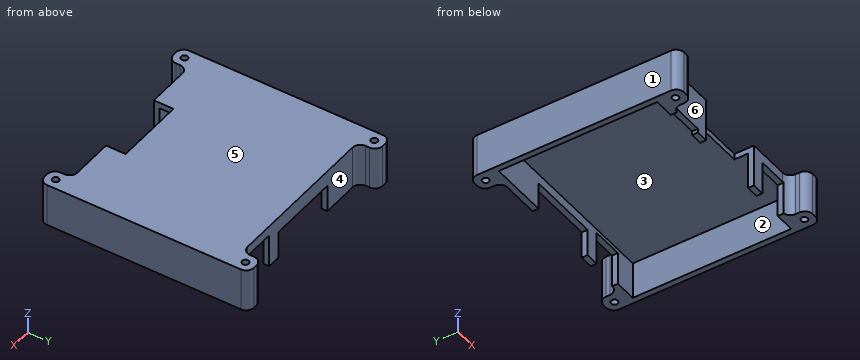
from build123d import *

# Parameters (mm, degrees)
SKETCH1_W                                  = 107
SKETCH1_H                                  = 87
BOSS_EXTRUDE1_DEPTH                        = 22
SKETCH2_W                                  = 10
SKETCH2_H                                  = 10
BOSS_EXTRUDE2_DEPTH                        = 22
MIRROR1_AT_THE_SECOND_PLANE_COPY_1_SKETC_W = 10
MIRROR1_AT_THE_SECOND_PLANE_COPY_1_SKETC_H = 10
MIRROR1_AT_THE_SECOND_PLANE_COPY_1_DEPTH   = 22
SKETCH3_W                                  = 101
SKETCH3_H                                  = 81
CUT_EXTRUDE1_DEPTH                         = 19
M3_CLEARANCE_HOLE1_D                       = 3.4
CUT_EXTRUDE2_REACH                         = 114.939
SKETCH6_W                                  = 16
SKETCH6_H                                  = 17
CUT_EXTRUDE6_REACH                         = 114.939
SKETCH12_W                                 = 16
SKETCH12_H                                 = 17
CUT_EXTRUDE3_REACH                         = 114.939
SKETCH8_W                                  = 37
SKETCH8_H                                  = 14
CUT_EXTRUDE4_REACH                         = 80.794
SKETCH9_W                                  = 36
SKETCH9_H                                  = 10
FILLET1_R                                  = 4
CUT_EXTRUDE5_REACH                         = 114.939
SKETCH11_W                                 = 16
SKETCH11_H                                 = 2
CUT_EXTRUDE5_DIRECTION_2_DEPTH             = 113.939142904


with BuildPart() as part:
    # Sketch1 → Boss-Extrude1 (new body)
    with BuildSketch(Plane.XY):
        Rectangle(SKETCH1_W, SKETCH1_H)
    extrude(amount=BOSS_EXTRUDE1_DEPTH)

    # Sketch2 → Boss-Extrude2 (add)
    with BuildSketch(Plane(origin=(0, 0, 0), x_dir=(-1, 0, 0), z_dir=(0, 0, -1))):
        with Locations((-48.5, -48.5)):
            Rectangle(SKETCH2_W, SKETCH2_H)
    boss_extrude2 = extrude(amount=-BOSS_EXTRUDE2_DEPTH)

    # Mirror1: Boss-Extrude2 across plane
    add(boss_extrude2.mirror(Plane.ZX))

    # Mirror1 at the second plane: Boss-Extrude2 across plane
    add(boss_extrude2.mirror(Plane(origin=(0, 0, 0), x_dir=(0, 0, 1), z_dir=(1, 0, 0))))

    # Mirror1 at the second plane copy 1 sketc → Mirror1 at the second plane copy 1 (add)
    with BuildSketch(Plane(origin=(0, 0, 0), x_dir=(1, 0, 0), z_dir=(0, 0, -1))):
        with Locations((-48.5, -48.5)):
            Rectangle(MIRROR1_AT_THE_SECOND_PLANE_COPY_1_SKETC_W, MIRROR1_AT_THE_SECOND_PLANE_COPY_1_SKETC_H)
    extrude(amount=-MIRROR1_AT_THE_SECOND_PLANE_COPY_1_DEPTH)

    # Sketch3 → Cut-Extrude1 (cut)
    with BuildSketch(Plane(origin=(0, 0, 0), x_dir=(-1, 0, 0), z_dir=(0, 0, -1))):
        Rectangle(SKETCH3_W, SKETCH3_H)
    extrude(amount=-CUT_EXTRUDE1_DEPTH, mode=Mode.SUBTRACT)

    # M3 Clearance Hole1 (through all)
    with Locations(Plane.XY.offset(22)):
        with Locations((-48.5, -48.5), (48.5, -48.5), (48.5, 48.5), (-48.5, 48.5)):
            Hole(M3_CLEARANCE_HOLE1_D / 2)

    # Sketch6 → Cut-Extrude2 (cut, up to next)
    with BuildSketch(Plane.XZ.offset(43.5), mode=Mode.PRIVATE) as cut_extrude2_sk1:
        with Locations((32.284998939, 8.5)):
            Rectangle(SKETCH6_W, SKETCH6_H)
    cut_extrude2_tool1 = extrude(cut_extrude2_sk1.sketch, amount=-CUT_EXTRUDE2_REACH, mode=Mode.PRIVATE) & part.part
    add(cut_extrude2_tool1.solids().sort_by_distance((32.284999, -43.5, 8.5))[0], mode=Mode.SUBTRACT)

    # Sketch12 → Cut-Extrude6 (cut, up to next)
    with BuildSketch(Plane(origin=(0, 43.5, 0), x_dir=(1, 0, 0), z_dir=(0, 1, 0)), mode=Mode.PRIVATE) as cut_extrude6_sk1:
        with Locations((31.284998153, -8.5)):
            Rectangle(SKETCH12_W, SKETCH12_H)
    cut_extrude6_tool1 = extrude(cut_extrude6_sk1.sketch, amount=-CUT_EXTRUDE6_REACH, mode=Mode.PRIVATE) & part.part
    add(cut_extrude6_tool1.solids().sort_by_distance((31.284998, 43.5, 8.5))[0], mode=Mode.SUBTRACT)

    # Sketch8 → Cut-Extrude3 (cut, up to next)
    with BuildSketch(Plane(origin=(0, 43.5, 0), x_dir=(1, 0, 0), z_dir=(0, 1, 0)), mode=Mode.PRIVATE) as cut_extrude3_sk1:
        with Locations((-2.036, -7)):
            Rectangle(SKETCH8_W, SKETCH8_H)
    cut_extrude3_tool1 = extrude(cut_extrude3_sk1.sketch, amount=-CUT_EXTRUDE3_REACH, mode=Mode.PRIVATE) & part.part
    add(cut_extrude3_tool1.solids().sort_by_distance((-2.036, 43.5, 7))[0], mode=Mode.SUBTRACT)

    # Sketch9 → Cut-Extrude4 (cut, up to next)
    with BuildSketch(Plane.XY.offset(22), mode=Mode.PRIVATE) as cut_extrude4_sk1:
        with Locations((-0.055943444, -38.5)):
            Rectangle(SKETCH9_W, SKETCH9_H)
    cut_extrude4_tool1 = extrude(cut_extrude4_sk1.sketch, amount=-CUT_EXTRUDE4_REACH, mode=Mode.PRIVATE) & part.part
    add(cut_extrude4_tool1.solids().sort_by_distance((-0.055943, -38.5, 22))[0], mode=Mode.SUBTRACT)

    # Fillet1
    fillet1_edges = [part.edges().sort_by_distance(p)[0] for p in [
        (43.5, -53.5, 11),
        (43.5, -43.5, 11),
        (53.5, -53.5, 11),
        (-53.5, -53.5, 11),
        (-43.5, -53.5, 11),
        (-43.5, -43.5, 11),
        (53.5, 53.5, 11),
        (43.5, 53.5, 11),
        (43.5, 43.5, 11),
        (-43.5, 53.5, 11),
        (-43.5, 43.5, 11),
        (-53.5, 53.5, 11),
    ]]
    fillet(fillet1_edges, radius=FILLET1_R)

    # Sketch11 → Cut-Extrude5 (cut, up to next)
    with BuildSketch(Plane.XZ.offset(43.5), mode=Mode.PRIVATE) as cut_extrude5_sk1:
        with Locations((-32.249997093, 1)):
            Rectangle(SKETCH11_W, SKETCH11_H)
    cut_extrude5_tool1 = extrude(cut_extrude5_sk1.sketch, amount=-CUT_EXTRUDE5_REACH, mode=Mode.PRIVATE) & part.part
    add(cut_extrude5_tool1.solids().sort_by_distance((-32.249997, -43.5, 1))[0], mode=Mode.SUBTRACT)

    # Sketch11 → Cut-Extrude5 direction 2 (cut)
    with BuildSketch(Plane.XZ.offset(43.5)):
        with Locations((-32.249997093, 1)):
            Rectangle(SKETCH11_W, SKETCH11_H)
    extrude(amount=CUT_EXTRUDE5_DIRECTION_2_DEPTH, mode=Mode.SUBTRACT)


solid = part.part
Source: CAD feature listing. Evaluate the final solid. Frame: model axes, mm. Face numbers are marked on the shaded views. A direction names the side the tool comes from. Give positions to 0.01 mm unless a question says otherwise; leave off trailing zeros. Write each loop counter-clockwise with the first axis right and the second up, starting at its lowest first coordinate (ties: lowest second). Pieces come first, ordered by that corner, then holes. Notation, with made-up numbers: (24, 31.5) - (71, 31.5) arc R25 ccw to (71, 66.5) - close; hole circle Ø8 at (63.5, 58.25). An arc over 180 degrees is marked (long way). Write item = value, one per line. Start each with the question number.
Q1. Cut plane A-A, the plane x = -37. Return loops of the section in (y, z), then the cut area to 3 significant figures.
Q2. Material intervals for probe 1 along Y at (x, z) = (-48.5, 13.25); probe 2 along X at (y, z) = (35, 10.75); probe 3 along Y at (x, z) = (-36.5, 14), sorted ascending.
Q3. Cut plane B-B, the plane z = 11.75. Give the number of separate pieces and of enclosed holes in the cut face, then the cut area to 3 significant figures.
Q4. Draft query along Y for the marked faces 3, 4, 5 and 6. Return one class per face: +Y half, -Y half, draft (parallel to the pull), parting line (faces both ways), or undercut.
Q5. Cut plane C-C, the plane y = -6.5. Return loops of the section in (x, z).
Q6. Pin query (flat end, axial travel): pin 1 Ø12 at (x, z) = (16, 19.5) entering from +Y; pin 2 Ø3.5 at (x, z) = (3.5, 20.5) entering from -Y; pin 3 Ø1.5 at (x, y) = (34.5, -42.5) entering from -Z. Return the tip coordinate at first contact, or that it passes through.
Q7. Reachability of the marked faces 1 and 2 from +Z, -Z, +X, -X, +Y, -Y: full face, straight path, thin tool, end or side. Return the list, or none.
Computed values:
q1.outline = (-43.5, 2) - (-40.5, 2) - (-40.5, 19) - (40.5, 19) - (40.5, 0) - (43.5, 0) - (43.5, 22) - (-43.5, 22) - close
q1.area = 369 mm²
q2.probe_1 = -53.5 to -50.2, -46.8 to -40.5, 40.5 to 46.8, 50.2 to 53.5
q2.probe_2 = -53.5 to -50.5, 50.5 to 53.5
q2.probe_3 = -43.5 to -40.5, 40.5 to 43.5
q3.separate_pieces = 4
q3.enclosed_holes = 4
q3.area = 1,160 mm²
q4.face_3 = undercut
q4.face_4 = +Y half
q4.face_5 = draft
q4.face_6 = -Y half
q5.outline = (-53.5, 0) - (-50.5, 0) - (-50.5, 19) - (50.5, 19) - (50.5, 0) - (53.5, 0) - (53.5, 22) - (-53.5, 22) - close
q6.pin_1 = 43.5
q6.pin_2 = -33.5
q6.pin_3 = 17
q7.face_1 = +Z, -Z, -X, +Y, -Y
q7.face_2 = -Z
